from build123d import *

# Parameters (mm, degrees)
BOSS_EXTRUDE1_DEPTH = 2
BOSS_EXTRUDE1_DRAFT = 45
SKETCH2_R           = 2.5
CUT_EXTRUDE1_DEPTH  = 114.154761278
SKETCH3_R           = 9
SKETCH3_R_2         = 7.5
BOSS_EXTRUDE2_DEPTH = 8
SKETCH4_W           = 2
SKETCH4_H           = 20
BOSS_EXTRUDE3_DEPTH = 10
SKETCH5_R           = 2
CUT_EXTRUDE2_DEPTH  = 10
CIRPATTERN1_COUNT   = 3


# Read off the part's stored shape, not the designer's step: Boss-Extrude1
with BuildPart() as part:
    # Boss-Extrude1 outline → Boss-Extrude1 (with draft: the straight prism first)
    with BuildSketch(Plane(origin=(0, 2, 0), x_dir=(1, 0, 0), z_dir=(0, 1, 0))):
        with BuildLine():
            ThreePointArc((-3.1, 77.938373091), (-67.549981495, 39), (-69.046611026, -36.284507794))
            Line((-69.046611026, -36.284507794), (-43.119219382, -21.315321248))
            Line((-43.119219382, -21.315321248), (-40.019219382, -26.684678752))
            Line((-40.019219382, -26.684678752), (-65.946611026, -41.653865297))
            ThreePointArc((-65.946611026, -41.653865297), (0, -78), (65.946611026, -41.653865297))
            Line((65.946611026, -41.653865297), (40.019219382, -26.684678752))
            Line((40.019219382, -26.684678752), (43.119219382, -21.315321248))
            Line((43.119219382, -21.315321248), (69.046611026, -36.284507794))
            ThreePointArc((69.046611026, -36.284507794), (67.549981495, 39), (3.1, 77.938373091))
            Line((3.1, 77.938373091), (3.1, 48))
            Line((3.1, 48), (-3.1, 48))
            Line((-3.1, 48), (-3.1, 77.938373091))
        make_face()
    extrude(amount=-BOSS_EXTRUDE1_DEPTH)
    # Boss-Extrude1: the draft: its side faces are tilted about the plane it starts from
    boss_extrude1_sides = [part.faces().sort_by_distance(p)[0] for p in [
        (67.549981495, 1, -39),
        (3.1, 1, -62.969186546),
        (0, 1, -48),
        (-3.1, 1, -62.969186546),
        (-67.549981495, 1, -39),
        (-56.082915204, 1, 28.799914521),
        (-41.569219382, 1, 24),
        (-52.982915204, 1, 34.169272025),
        (0, 1, 78),
        (52.982915204, 1, 34.169272025),
        (41.569219382, 1, 24),
        (56.082915204, 1, 28.799914521),
    ]]
    draft(boss_extrude1_sides, Plane(origin=(0, 2, 0), x_dir=(1, 0, 0), z_dir=(0, 1, 0)), BOSS_EXTRUDE1_DRAFT)

    # Sketch2 → Cut-Extrude1 (cut, through all)
    with BuildSketch(Plane(origin=(0, 2, 0), x_dir=(1, 0, 0), z_dir=(0, 1, 0))):
        with Locations(Location((0, 0, 0), (0, 0, 270))):
            Circle(SKETCH2_R)
    extrude(amount=-CUT_EXTRUDE1_DEPTH, mode=Mode.SUBTRACT)

    # Sketch3 → Boss-Extrude2 (add)
    with BuildSketch(Plane(origin=(0, 2, 0), x_dir=(1, 0, 0), z_dir=(0, 1, 0))):
        with Locations(Location((0, 0, 0), (0, 0, 270))):
            Circle(SKETCH3_R)
        with Locations(Location((0, 0, 0), (0, 0, 270))):
            Circle(SKETCH3_R_2, mode=Mode.SUBTRACT)
    extrude(amount=BOSS_EXTRUDE2_DEPTH)

    # Sketch4 → Boss-Extrude3 (add)
    with BuildSketch(Plane.XZ):
        Polygon((42.751270189, 25.952627944), (60.071778265, 35.952627944), (59.071778265, 37.684678752), (41.751270189, 27.684678752), align=None)
        Polygon((43.851270189, 24.047372056), (61.171778265, 34.047372056), (62.171778265, 32.315321248), (44.851270189, 22.315321248), align=None)
        with Locations((2.1, -60)):
            Rectangle(SKETCH4_W, SKETCH4_H)
        with Locations((-2.1, -60)):
            Rectangle(SKETCH4_W, SKETCH4_H)
        Polygon((-44.851270189, 22.315321248), (-62.171778265, 32.315321248), (-61.171778265, 34.047372056), (-43.851270189, 24.047372056), align=None)
        Polygon((-42.751270189, 25.952627944), (-60.071778265, 35.952627944), (-59.071778265, 37.684678752), (-41.751270189, 27.684678752), align=None)
    extrude(amount=BOSS_EXTRUDE3_DEPTH)

    # Sketch5 → Cut-Extrude2 (cut)
    with BuildSketch(Plane(origin=(3.1, 0, 0), x_dir=(0, 0, -1), z_dir=(1, 0, 0))):
        with Locations((55, -5)):
            Circle(SKETCH5_R)
    cut_extrude2 = extrude(amount=-CUT_EXTRUDE2_DEPTH, mode=Mode.SUBTRACT)

    # CirPattern1: Cut-Extrude2 ×3 about axis
    cirpattern1_axis = Axis((0, 10, 0), (0, -1, 0))
    for i in range(1, CIRPATTERN1_COUNT):
        add(cut_extrude2.rotate(cirpattern1_axis, i * 360 / CIRPATTERN1_COUNT), mode=Mode.SUBTRACT)


solid = part.part
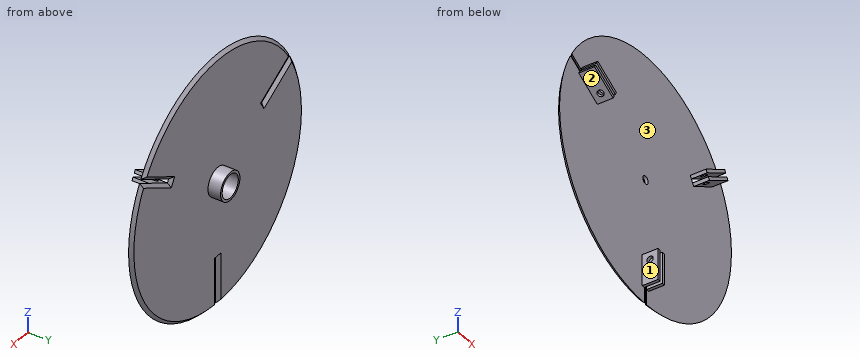
Verification items for the finished model (mm, model axes). Face numbers are marked on the shaded views. A direction names the side the tool comes from. Coordinates: 2 decimals unless noted, no trailing zeros. Write each loop counter-clockwise with the first axis right and the second up, starting at its lowest first coordinate (ties: lowest second). Pieces come first, ordered by that corner, then holes. Notation, with made-up numbers: (21, 27) -> (35, 27) arc R13 ccw to (35, 37) -> close; hole circle Ø8 at (17.25, 88.5). An arc over 180 degrees is marked (long way). One line per item, written item: value. Start each with the question number.
Q1. Access from +Z, -Z, +X, -X, +Y, -Y to the whole of each face (thin tool, end or side, straight path). Record for the marked faces 1, 2 and 3.
Q2. Cross-section at A-A on z = 0. Enter the section's corners in (x, y).
Q3. Thickness scan on L1, parallel to X at y = 8.25, z = 0; L2, parallel to Y at x = 6.5, z = 50; L3, parallel to X at y = 0.95, z = 0. Record the ranges inside material, lowest first. Write a range as from..to.
Q4. Go/stop test with flat-tipped pins: P1, Ø6.5, axis at y = -5, z = -55, coming from the +X side; P2, Ø5, axis at y = -3, z = -61, coming from the -X side; P3, Ø2, axis at x = 2, y = -6, coming from the -Z side. Record where each tip stops, or that it passes through.
Q5. Cross-section at B-B on y = 7. Enter the section's corners in (x, z), and give its area (3 significant figures).
Q6. Cross-section at C-C on z = -55. State how many separate pieces and enclosed holes the cut face has, and give its area (3 significant figures).
Checked values:
1. face 1: +Z, -Z, -X, -Y
1. face 2: -Z, -X, -Y
1. face 3: -Y
2. outline: (-80, 0) -> (-2.5, 0) -> (-2.5, 2) -> (-7.5, 2) -> (-7.5, 10) -> (-9, 10) -> (-9, 2) -> (-78, 2) -> close; (2.5, 0) -> (80, 0) -> (78, 2) -> (9, 2) -> (9, 10) -> (7.5, 10) -> (7.5, 2) -> (2.5, 2) -> close
3. L1: x = -9..-7.5, 7.5..9
3. L2: y = 0..2
3. L3: x = -79.05..-2.5, 2.5..79.05
4. P1: stops at x = 3.1
4. P2: stops at x = -3.1
4. P3: stops at z = -70
5. outline: circle Ø18 at (0, 0); hole circle Ø15 at (0, 0)
5. area: 77.8 mm²
6. separate pieces: 4
6. enclosed holes: 0
6. area: 242 mm²
